Could you check a few things on this model? Use its own coordinates, in mm. Face numbers are marked on the shaded views. A direction names the side the tool comes from. Round coordinates to 2 decimals unless told otherwise and drop trailing zeros. Loops run counter-clockwise (first coordinate to the right, second up) from the corner with the lowest first, then second, coordinate; pieces in that order, holes last. Notation, with made-up numbers: (-7, 76.25) -> (47, 76.25) arc R5 cw to (47, 84.25) -> close; hole circle Ø10 at (84, -17). An arc over 180 degrees is marked (long way). Write each question's results on one line, items separated by ' | '. Start each with the question number.
1) Imagine slicing it at A-A, the plane x = 13.75. List the corners of the cut face in (y, z) for me, plus the area to 3 significant figures.
2) For P1, Ø3, axis at x = 9, y = -1.5, coming from the -Z side; P2, Ø3, axis at y = 0, z = -6.5, coming from the +X side; P3, Ø1.5, axis at x = -0.5, y = 0.5, coming from the -Z side, each with a flat end and sliding along its axis, tell me the tip position at first contact or that it passes through.
3) We'd pull the mould along Y, two halves only. Please class the marked faces 4, 5 and 6: pulls with the +Y half, pulls with the -Y half, needs draft (parallel to the pull), parting line crosses it, or undercut.
4) Imagine slicing it at D-D, the plane x = 0. List the corners of the cut face in (y, z) for me.
5) If I drill on probe 1 along Y at (x, z) = (6.5, 0); probe 2 along X at (y, z) = (1, 0.5); probe 3 along X at (y, z) = (-0.25, -3.75), over which ranges is the centre line in solid material (lowest first)?
6) Imagine slicing it at C-C, the plane y = 0. List the corners of the cut face in (x, z) for me.
7) Which directions (+Z, -Z, +X, -X, +Y, -Y) give clear straight access to the entire face, cutting with the end or side of a thin tool? Please do the marked faces 1, 2 and 3.
8) Imagine slicing it at B-B, the plane z = -14.5. List the corners of the cut face in (x, y) for me.
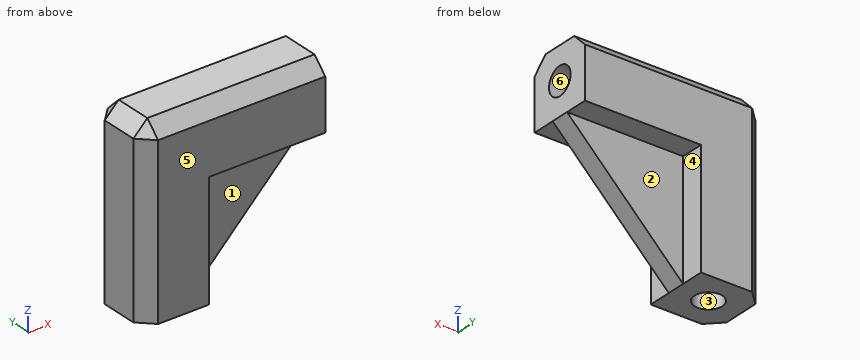
from build123d import *

# Parameters (mm, degrees)
BOSS_EXTRUDE1_DEPTH = 3.5
SKETCH2_R           = 1.5
CUT_EXTRUDE1_DEPTH  = 14
SKETCH3_R           = 1.5
CUT_EXTRUDE2_DEPTH  = 14
BOSS_EXTRUDE2_DEPTH = 1
CHAMFER1_SIZE       = 1.5


with BuildPart() as part:
    # Sketch1 → Boss-Extrude1 (new, symmetric)
    with BuildSketch(Plane(origin=(0, 0, 0), x_dir=(1, 0, 0), z_dir=(0, 1, 0))):
        Polygon((-3.5, 16), (-3.5, -3.5), (16, -3.5), (16, 3.5), (3.5, 3.5), (3.5, 16), align=None)
    extrude(amount=BOSS_EXTRUDE1_DEPTH, both=True)

    # Sketch2 → Cut-Extrude1 (cut)
    with BuildSketch(Plane(origin=(0, 0, -16), x_dir=(-1, 0, 0), z_dir=(0, 0, -1))):
        Circle(SKETCH2_R)
    extrude(amount=-CUT_EXTRUDE1_DEPTH, mode=Mode.SUBTRACT)

    # Sketch3 → Cut-Extrude2 (cut)
    with BuildSketch(Plane(origin=(16, 0, 0), x_dir=(0, 0, -1), z_dir=(1, 0, 0))):
        Circle(SKETCH3_R)
    extrude(amount=-CUT_EXTRUDE2_DEPTH, mode=Mode.SUBTRACT)

    # Sketch4 → Boss-Extrude2 (add, symmetric)
    with BuildSketch(Plane(origin=(0, 0, 0), x_dir=(1, 0, 0), z_dir=(0, 1, 0))):
        Polygon((3.5, 16), (16, 3.5), (3.5, 3.5), align=None)
    extrude(amount=BOSS_EXTRUDE2_DEPTH, both=True)

    # Chamfer1
    chamfer1_edges = [part.edges().sort_by_distance(p)[0] for p in [
        (-3.5, 0, 3.5),
        (6.25, 3.5, 3.5),
        (6.25, -3.5, 3.5),
        (-3.5, -3.5, -6.25),
        (-3.5, 3.5, -6.25),
    ]]
    chamfer(chamfer1_edges, length=CHAMFER1_SIZE)


solid = part.part
Checked values:
1) outline: (-3.5, -3.5) -> (-1, -3.5) -> (-1, -5.75) -> (1, -5.75) -> (1, -3.5) -> (3.5, -3.5) -> (3.5, 2) -> (2, 3.5) -> (-2, 3.5) -> (-3.5, 2) -> close; hole circle Ø3 at (0, 0) | area: 44.2 mm^2
2) P1: z = -11.91 | P2: x = 14.5 | P3: z = -2
3) face 4: needs draft | face 5: pulls with the -Y half | face 6: undercut
4) outline: (-3.5, -16) -> (-1.5, -16) -> (-1.5, -2) -> (1.5, -2) -> (1.5, -16) -> (3.5, -16) -> (3.5, 2) -> (2, 3.5) -> (-2, 3.5) -> (-3.5, 2) -> close
5) probe 1: -3.5 to -1.5, 1.5 to 3.5 | probe 2: -3.5 to 2 | probe 3: -3.5 to -1.48, 1.48 to 15.75
6) outline: (-3.5, -16) -> (-1.5, -16) -> (-1.5, -2) -> (1.5, -2) -> (1.5, -16) -> (3.5, -16) -> (16, -3.5) -> (16, -1.5) -> (2, -1.5) -> (2, 1.5) -> (16, 1.5) -> (16, 3.5) -> (-2, 3.5) -> (-3.5, 2) -> close
7) face 1: -Z, +X, -Y | face 2: -Z, +X, +Y | face 3: -Z
8) outline: (-3.5, -2) -> (-2, -3.5) -> (3.5, -3.5) -> (3.5, -1) -> (5, -1) -> (5, 1) -> (3.5, 1) -> (3.5, 3.5) -> (-2, 3.5) -> (-3.5, 2) -> close; hole circle Ø3 at (0, 0)
